from build123d import *

# Parameters (mm, degrees)
BOSS_EXTRUDE1_DEPTH = 15
SHELL1_T            = 2
BOSS_EXTRUDE2_DEPTH = 15
SKETCH4_R           = 2
CUT_EXTRUDE3_DEPTH  = 17
SKETCH5_W           = 37.9
SKETCH5_H           = 37.3
BOSS_EXTRUDE3_DEPTH = 10
SKETCH8_W           = 35.9
SKETCH8_H           = 35.3
CUT_EXTRUDE4_DEPTH  = 1.6
SKETCH9_W           = 19.2
SKETCH9_H           = 30
BOSS_EXTRUDE5_DEPTH = 13.6
SKETCH11_W          = 17.2
SKETCH11_H          = 28
CUT_EXTRUDE7_DEPTH  = 1.6
CUT_EXTRUDE8_DEPTH  = 2


# Read off the part's stored shape, not the designer's step: Boss-Extrude2
with BuildPart() as part:
    # Sketch2 → Boss-Extrude1 (new body)
    with BuildSketch(Plane(origin=(0, 0, 0), x_dir=(1, 0, 0), z_dir=(0, 1, 0))):
        with BuildLine():
            Line((-29.057488174, 43.856363161), (-21.094956582, -19.84388958))
            ThreePointArc((-21.094956582, -19.84388958), (-17.790203447, -26.100323992), (-11.172177815, -28.603542234))
            Line((-11.172177815, -28.603542234), (11.172177815, -28.603542234))
            ThreePointArc((11.172177815, -28.603542234), (17.790203447, -26.100323992), (21.094956582, -19.84388958))
            Line((21.094956582, -19.84388958), (29.057488174, 43.856363161))
            ThreePointArc((29.057488174, 43.856363161), (27.625040268, 50.380107319), (22.404958564, 54.546867672))
            ThreePointArc((22.404958564, 54.546867672), (0, 58.313921904), (-22.404958564, 54.546867672))
            ThreePointArc((-22.404958564, 54.546867672), (-27.625040268, 50.380107319), (-29.057488174, 43.856363161))
        make_face()
    extrude(amount=BOSS_EXTRUDE1_DEPTH)

    # Shell1
    shell1_openings = [part.faces().sort_by_distance(p)[0] for p in [
        (0, 15, -16.825507136),
    ]]
    offset(amount=SHELL1_T, openings=shell1_openings, kind=Kind.INTERSECTION)

    # Boss-Extrude2 outline → Boss-Extrude2 (add)
    with BuildSketch(Plane(origin=(0, 0, 0), x_dir=(1, 0, 0), z_dir=(0, 1, 0))):
        with BuildLine():
            ThreePointArc((11.172177815, -28.603542234), (17.478052637, -26.364724021), (20.960385979, -20.65073078))
            ThreePointArc((20.960385979, -20.65073078), (14.125965093, -22.239021953), (11.172177815, -28.603542234))
        make_face()
        with BuildLine():
            ThreePointArc((22.404958564, 54.546867672), (22.805580573, 46.686663567), (28.769287815, 41.550760286))
            Line((28.769287815, 41.550760286), (29.057488174, 43.856363161))
            ThreePointArc((29.057488174, 43.856363161), (27.625040268, 50.380107319), (22.404958564, 54.546867672))
        make_face()
        with BuildLine():
            ThreePointArc((-11.172177815, -28.603542234), (-14.125965093, -22.239021953), (-20.960385978, -20.65073078))
            ThreePointArc((-20.960385978, -20.65073078), (-17.478052637, -26.364724021), (-11.172177815, -28.603542234))
        make_face()
        with BuildLine():
            Line((-29.057488174, 43.856363161), (-28.769287815, 41.550760286))
            ThreePointArc((-28.769287815, 41.550760286), (-22.805580573, 46.686663567), (-22.404958564, 54.546867672))
            ThreePointArc((-22.404958564, 54.546867672), (-27.625040268, 50.380107319), (-29.057488174, 43.856363161))
        make_face()
    extrude(amount=BOSS_EXTRUDE2_DEPTH)

    # Sketch4 → Cut-Extrude3 (cut)
    with BuildSketch(Plane(origin=(0, 15, 0), x_dir=(1, 0, 0), z_dir=(0, 1, 0))):
        with Locations(Location((-26.203765036, 48.932847943, 0), (0, 0, 270))):
            Circle(SKETCH4_R)
        with Locations(Location((-17.279655559, -24.618760567, 0), (0, 0, 270))):
            Circle(SKETCH4_R)
        with Locations(Location((17.279655559, -24.618760567, 0), (0, 0, 270))):
            Circle(SKETCH4_R)
        with Locations(Location((26.203765036, 48.932847943, 0), (0, 0, 270))):
            Circle(SKETCH4_R)
    extrude(amount=-CUT_EXTRUDE3_DEPTH, mode=Mode.SUBTRACT)

    # Sketch5 → Boss-Extrude3 (add)
    with BuildSketch(Plane(origin=(-2.134010057, 0, 0), x_dir=(1, 0, 0), z_dir=(0, 1, 0))):
        with Locations((1.95, 28.65)):
            Rectangle(SKETCH5_W, SKETCH5_H)
    extrude(amount=BOSS_EXTRUDE3_DEPTH)

    # Sketch8 → Cut-Extrude4 (cut)
    with BuildSketch(Plane(origin=(48.898344446, 10, 0), x_dir=(1, 0, 0), z_dir=(0, 1, 0))):
        with Locations((-49.05, 28.65)):
            Rectangle(SKETCH8_W, SKETCH8_H)
    extrude(amount=-CUT_EXTRUDE4_DEPTH, mode=Mode.SUBTRACT)

    # Sketch9 → Boss-Extrude5 (add)
    with BuildSketch(Plane(origin=(0, 0, 0), x_dir=(1, 0, 0), z_dir=(0, 1, 0))):
        with Locations((0.1, -13.603542234)):
            Rectangle(SKETCH9_W, SKETCH9_H)
    extrude(amount=BOSS_EXTRUDE5_DEPTH)

    # Sketch11 → Cut-Extrude7 (cut)
    with BuildSketch(Plane(origin=(0, 13.6, 0), x_dir=(1, 0, 0), z_dir=(0, 1, 0))):
        with Locations((0.1, -14.603542234)):
            Rectangle(SKETCH11_W, SKETCH11_H)
    extrude(amount=-CUT_EXTRUDE7_DEPTH, mode=Mode.SUBTRACT)

    # Sketch12 → Cut-Extrude8 (cut)
    with BuildSketch(Plane.XY.offset(30.603542234)):
        with BuildLine():
            Line((-4.15, 15), (4.35, 15))
            ThreePointArc((4.35, 15), (4.110077828, 14.306431155), (3.45, 13.985654515))
            Line((3.45, 13.985654515), (-3.25, 13.821910042))
            ThreePointArc((-3.25, 13.821910042), (-3.943990419, 14.224558918), (-4.15, 15))
        make_face()
    extrude(amount=-CUT_EXTRUDE8_DEPTH, mode=Mode.SUBTRACT)


solid = part.part
CAD build for the part. Positions are in the model's coordinates, mm. A direction names the side the tool comes from. Round coordinates to 2 decimals unless told otherwise and drop trailing zeros. Loops run counter-clockwise (first coordinate to the right, second up) from the corner with the lowest first, then second, coordinate; pieces in that order, holes last. Notation, with made-up numbers: (52, 37) - (66, 37) arc R17 cw to (66, 69) - close; hole circle Ø11 at (1, 81.5). An arc over 180 degrees is marked (long way). Put each result on its own line as item: value.
1. Slice it at B-B on z = 10. List the corners of the cut face in (x, y).
Geometry check:
outline: (-24.34, -2) - (24.34, -2) - (24.34, 15) - (22.33, 15) - (22.33, 0) - (9.7, 0) - (9.7, 13.6) - (8.7, 13.6) - (8.7, 12) - (-8.5, 12) - (-8.5, 13.6) - (-9.5, 13.6) - (-9.5, 0) - (-22.33, 0) - (-22.33, 15) - (-24.34, 15) - close
2. Two-plate mould, pull along Z, no slides. Class faces 1 (the flat face through (-19.134, 5, -28)), 2 (the cylindrical face through (0.329, 6.381, -60.313)), 3 (the flat face through (0, 5, -10)), 4 (the flat face through (-26, 15, -15)): released by +Z, released by -Z, zero draft, split by the parting line, or undercut.
Geometry check:
face 1: undercut
face 2: released by -Z
face 3: undercut
face 4: zero draft
3. Pin check, flat tips, straight feed: P1, Ø6, axis at x = 4, y = 0, coming from the -Z side; P2, Ø1, axis at y = 9, z = -3.5, coming from the +X side; P3, Ø1.3, axis at y = 12.5, z = 19, coming from the +X side. Stop position of each tip, or through.
Geometry check:
P1: z = -60.31
P2: x = 26.09
P3: x = 23.3
4. 3-axis set-ups, long thin cutter, end or side, ignore diameter. For faces 5 (the cylindrical face through (-14.05, 7.4, 22.3)), 6 (the cylindrical face through (16.063, 6.619, 23.032)): which of +Z, -Z, +X, -X, +Y, -Y reach the whole face in a straight line?
Geometry check:
face 5: +Y
face 6: +Y, -Y
5. Slice it at A-A on y = 1. Give the number of separate pieces and of enclosed holes in the cut face, and give its area (3 significant figures).
Geometry check:
separate pieces: 2
enclosed holes: 5
area: 2,670 mm²
6. Wall check: line 1 (Z direction, x = 11, y = 7.75); line 2 (Z direction, x = -5.5, y = 2.5); line 3 (X direction, y = 3, z = -44). Give the ranges that are in metal, low to high.
Geometry check:
line 1: -59.45 to -57.43, -47.3 to -10, 28.6 to 30.6
line 2: -60.1 to -58.09, -47.3 to -10, -1.4 to 30.6
line 3: -31.08 to -24.73, -19.13 to 18.77, 24.73 to 31.08
7. Slice it at C-C on x = 13. List the corners of the cut face in (y, z).
Geometry check:
outline: (-2, -59.11) - (15, -59.11) - (15, -57.07) - (0, -57.07) - (0, -47.3) - (10, -47.3) - (10, -46.3) - (8.4, -46.3) - (8.4, -11) - (10, -11) - (10, -10) - (0, -10) - (0, 23.36) - (15, 23.36) - (15, 30.46) - (-2, 30.46) - close
8. Slice it at D-D on z = -3. List the corners of the cut face in (x, y), and give its area (3 significant figures).
Geometry check:
outline: (-25.97, -2) - (25.97, -2) - (25.97, 15) - (23.95, 15) - (23.95, 0) - (-23.95, 0) - (-23.95, 15) - (-25.97, 15) - close
area: 164 mm²
